The listing builds one solid part. Answer for the finished solid, in the listing's coordinates (mm). A direction names the side the tool comes from. Coordinates: 2 decimals unless noted, no trailing zeros. Order: outer loops, then holes, each group sorted by start corner. A loop starts at its lowest first (then second) coordinate and runs counter-clockwise, first axis right, second up. Notation, with made-up numbers: (-17.5, 89.25) -> (-1.5, 89.25) arc R7 ccw to (-1.5, 94.25) -> close; hole circle Ø7 at (42.5, 6). An arc over 180 degrees is marked (long way). Answer in a Markdown table with one row per item.
```python
from build123d import *

# Parameters (mm, degrees)
SKETCH1_W           = 25
SKETCH1_H           = 40
BOSS_EXTRUDE1_DEPTH = 10
SKETCH2_R           = 1.5
CUT_EXTRUDE1_DEPTH  = 34.541019662
SKETCH4_R           = 1.5
CUT_EXTRUDE3_DEPTH  = 34.541019662
SKETCH6_W           = 2
SKETCH6_H           = 2
CUT_EXTRUDE4_DEPTH  = 44.084219849


with BuildPart() as part:
    # Sketch1 → Boss-Extrude1 (new body)
    with BuildSketch(Plane(origin=(0, 0, 0), x_dir=(1, 0, 0), z_dir=(0, 1, 0))):
        Rectangle(SKETCH1_W, SKETCH1_H)
    extrude(amount=BOSS_EXTRUDE1_DEPTH)

    # Sketch2 → Cut-Extrude1 (cut, through all)
    with BuildSketch(Plane(origin=(12.5, 0, 0), x_dir=(0, 0, -1), z_dir=(1, 0, 0))):
        with Locations((10, 5)):
            Circle(SKETCH2_R)
    extrude(amount=-CUT_EXTRUDE1_DEPTH, mode=Mode.SUBTRACT)

    # Sketch4 → Cut-Extrude3 (cut, through all)
    with BuildSketch(Plane.ZY.offset(12.5)):
        with Locations((5, 5)):
            Circle(SKETCH4_R)
    extrude(amount=-CUT_EXTRUDE3_DEPTH, mode=Mode.SUBTRACT)

    # Sketch6 → Cut-Extrude4 (cut, through all)
    with BuildSketch(Plane.XY.offset(20)):
        with Locations((0, 5)):
            Rectangle(SKETCH6_W, SKETCH6_H)
    extrude(amount=-CUT_EXTRUDE4_DEPTH, mode=Mode.SUBTRACT)


solid = part.part
```
(1) Which of the six approach directions +Z, -Z, +X, -X, +Y, -Y give full straight-line access (tool end or side, diameter ignored) to faces 1 (the flat face through (0, 4, -15)), 2 (the flat face through (-0.2, 3.8, 20))?
Check values:
| item | result |
|---|---|
| face 1 | +Z, -Z |
| face 2 | +Z, +X, -X, +Y, -Y |
(2) A cutting plane is placed at C-C, the plane x = -8.5. Determine the outline of the cut face in (y, z), then the cut area to 3 significant figures.
Check values:
| item | result |
|---|---|
| outline | (0, -20) -> (10, -20) -> (10, 20) -> (0, 20) -> close; hole circle Ø3 at (5, -10); hole circle Ø3 at (5, 5) |
| area | 386 mm² |
(3) A cutting plane is placed at D-D, the plane z = -15.5. Determine the outline of the cut face in (x, y), then the cut area to 3 significant figures.
Check values:
| item | result |
|---|---|
| outline | (-12.5, 0) -> (12.5, 0) -> (12.5, 10) -> (-12.5, 10) -> close; hole (-1, 4) -> (1, 4) -> (1, 6) -> (-1, 6) -> close |
| area | 246 mm² |
(4) Find the intervals of material crossed by line 1 along Z through (x, y) = (1.5, 6); line 2 along Z through (x, y) = (-7.25, 5); line 3 along Y through (x, z) = (-5, 5), in increasing order. Write a range as from..to.
Check values:
| item | result |
|---|---|
| line 1 | -20..-11.12, -8.88..3.88, 6.12..20 |
| line 2 | -20..-11.5, -8.5..3.5, 6.5..20 |
| line 3 | 0..3.5, 6.5..10 |
(5) For a pull along Y with two mould halves and no side action, classify faces 3 (the flat face through (-0.2, 3.8, -20)), 4 (the flat face through (0, 0, 0)), 5 (the cylindrical face through (0.175, 6.487, -9.805)), 6 (the flat face through (0, 10, 0)) as released by +Y, released by -Y, zero draft, split by the parting line, or undercut.
Check values:
| item | result |
|---|---|
| face 3 | zero draft |
| face 4 | released by -Y |
| face 5 | undercut |
| face 6 | released by +Y |
(6) A cutting plane is placed at B-B, the plane z = 5. Determine the outline of the cut face in (x, y), then the cut area to 3 significant figures.
Check values:
| item | result |
|---|---|
| outline | (-12.5, 0) -> (12.5, 0) -> (12.5, 3.5) -> (-12.5, 3.5) -> close; (-12.5, 6.5) -> (12.5, 6.5) -> (12.5, 10) -> (-12.5, 10) -> close |
| area | 175 mm² |
(7) A flat-ended cylindrical pin translates along its axis: pin 1 (2.5 mm diameter, centred on y = 5, z = 5, fed in from -X). Find the tip coordinate at first contact, or state that the pin passes through.
Check values:
| item | result |
|---|---|
| pin 1 | through |
(8) A cutting plane is placed at A-A, the plane y = 5. Determine the outline of the cut face in (x, z).
Check values:
| item | result |
|---|---|
| outline | (-12.5, -20) -> (-1, -20) -> (-1, -11.5) -> (-12.5, -11.5) -> close; (-12.5, -8.5) -> (-1, -8.5) -> (-1, 3.5) -> (-12.5, 3.5) -> close; (-12.5, 6.5) -> (-1, 6.5) -> (-1, 20) -> (-12.5, 20) -> close; (1, -20) -> (12.5, -20) -> (12.5, -11.5) -> (1, -11.5) -> close; (1, -8.5) -> (12.5, -8.5) -> (12.5, 3.5) -> (1, 3.5) -> close; (1, 6.5) -> (12.5, 6.5) -> (12.5, 20) -> (1, 20) -> close |
